from build123d import *

# Parameters (mm, degrees)
BOSS_EXTRUDE1_DEPTH = 36
BOSS_EXTRUDE2_DEPTH = 12
SKETCH1_6_W         = 12
SKETCH1_6_H         = 48
SKETCH1_6_W_2       = 25
SKETCH1_6_W_3       = 23
SKETCH1_6_H_2       = 12
BOSS_EXTRUDE4_DEPTH = 24
SKETCH1_8_W         = 25
SKETCH1_8_H         = 12
SKETCH1_8_H_2       = 48
SKETCH1_8_W_2       = 23
CUT_EXTRUDE2_DEPTH  = 12
BOSS_EXTRUDE5_START = 24
SKETCH1_10_W        = 23
SKETCH1_10_H        = 12
SKETCH1_10_W_2      = 12
SKETCH1_10_W_3      = 25
BOSS_EXTRUDE5_DEPTH = 12
CUT_EXTRUDE3_DEPTH  = 12
FILLET1_R           = 5


with BuildPart() as part:
    # Sketch1 → Boss-Extrude1 (new body)
    with BuildSketch(Plane(origin=(0, 0, 0), x_dir=(0, 1, 0), z_dir=(0, 0, 1))):
        with BuildLine():
            Line((36, -30), (27, -30))
            ThreePointArc((27, -30), (45, -48), (63, -30))
            ThreePointArc((63, -30), (57.727922061, -17.272077939), (45, -12))
            Line((45, -12), (45, -21))
            ThreePointArc((45, -21), (51.363961031, -23.636038969), (54, -30))
            ThreePointArc((54, -30), (45, -39), (36, -30))
        make_face()
        with BuildLine():
            ThreePointArc((39, -13.029437252), (30.303061543, -19.607695155), (27, -30))
            Line((27, -30), (36, -30))
            ThreePointArc((36, -30), (36.784161637, -26.325765386), (39, -23.291796068))
            Line((39, -23.291796068), (39, -13.029437252))
        make_face()
        with BuildLine():
            ThreePointArc((45, -12), (41.956164383, -12.259225926), (39, -13.029437252))
            Line((39, -13.029437252), (39, -23.291796068))
            ThreePointArc((39, -23.291796068), (41.788601192, -21.592448769), (45, -21))
            Line((45, -21), (45, -12))
        make_face()
        with BuildLine():
            ThreePointArc((39, 13.029437252), (30.303061543, 19.607695155), (27, 30))
            Line((27, 30), (27, 18))
            Line((27, 18), (27, -30))
            ThreePointArc((27, -30), (30.303061543, -19.607695155), (39, -13.029437252))
            Line((39, -13.029437252), (39, 13.029437252))
        make_face()
        with BuildLine():
            Line((36, 30), (27, 30))
            ThreePointArc((27, 30), (30.303061543, 19.607695155), (39, 13.029437252))
            Line((39, 13.029437252), (39, 23.291796068))
            ThreePointArc((39, 23.291796068), (36.784161637, 26.325765386), (36, 30))
        make_face()
        with BuildLine():
            ThreePointArc((63, 30), (45, 48), (27, 30))
            Line((27, 30), (36, 30))
            ThreePointArc((36, 30), (45, 39), (54, 30))
            ThreePointArc((54, 30), (51.363961031, 23.636038969), (45, 21))
            Line((45, 21), (45, 12))
            ThreePointArc((45, 12), (57.727922061, 17.272077939), (63, 30))
        make_face()
        with BuildLine():
            Line((39, 23.291796068), (39, 13.029437252))
            ThreePointArc((39, 13.029437252), (41.956164383, 12.259225926), (45, 12))
            Line((45, 12), (45, 21))
            ThreePointArc((45, 21), (41.788601192, 21.592448769), (39, 23.291796068))
        make_face()
    extrude(amount=BOSS_EXTRUDE1_DEPTH)

    # Sketch1_4 → Boss-Extrude2 (add)
    with BuildSketch(Plane(origin=(0, 0, 0), x_dir=(0, 1, 0), z_dir=(0, 0, 1))):
        with BuildLine():
            ThreePointArc((45, 12), (41.956164383, 12.259225926), (39, 13.029437252))
            Line((39, 13.029437252), (39, -13.029437252))
            ThreePointArc((39, -13.029437252), (41.956164383, -12.259225926), (45, -12))
            Line((45, -12), (45, 12))
        make_face()
        with BuildLine():
            Line((63, -30), (63, 30))
            ThreePointArc((63, 30), (57.727922061, 17.272077939), (45, 12))
            Line((45, 12), (45, -12))
            ThreePointArc((45, -12), (57.727922061, -17.272077939), (63, -30))
        make_face()
    extrude(amount=BOSS_EXTRUDE2_DEPTH)

    # Sketch1_6 → Boss-Extrude4 (add)
    # profile 1 of 8: a face of its own
    with BuildSketch(Plane(origin=(0, 0, 0), x_dir=(0, 1, 0), z_dir=(0, 0, 1))):
        with Locations((-2, -6)):
            Rectangle(SKETCH1_6_W, SKETCH1_6_H)
    # profile 2 of 8: a face of its own
    with BuildSketch(Plane(origin=(0, 0, 0), x_dir=(0, 1, 0), z_dir=(0, 0, 1))):
        with Locations((-20.5, -6)):
            Rectangle(SKETCH1_6_W_2, SKETCH1_6_H)
        with BuildLine():
            Line((-28, -8), (-28, 1))
            ThreePointArc((-28, 1), (-20, 9), (-12, 1))
            Line((-12, 1), (-12, -8))
            ThreePointArc((-12, -8), (-20, -16), (-28, -8))
        make_face(mode=Mode.SUBTRACT)
    # profile 3 of 8: a face of its own
    with BuildSketch(Plane(origin=(0, 0, 0), x_dir=(0, 1, 0), z_dir=(0, 0, 1))):
        with Locations((15.5, -6)):
            Rectangle(SKETCH1_6_W_3, SKETCH1_6_H)
    # profile 4 of 8: a face of its own
    with BuildSketch(Plane(origin=(0, 0, 0), x_dir=(0, 1, 0), z_dir=(0, 0, 1))):
        with Locations((-39, -6)):
            Rectangle(SKETCH1_6_W, SKETCH1_6_H)
    # profile 5 of 8: a face of its own
    with BuildSketch(Plane(origin=(0, 0, 0), x_dir=(0, 1, 0), z_dir=(0, 0, 1))):
        with Locations((15.5, 24)):
            Rectangle(SKETCH1_6_W_3, SKETCH1_6_H_2)
    # profile 6 of 8: a face of its own
    with BuildSketch(Plane(origin=(0, 0, 0), x_dir=(0, 1, 0), z_dir=(0, 0, 1))):
        with Locations((-2, 24)):
            Rectangle(SKETCH1_6_W, SKETCH1_6_H_2)
    # profile 7 of 8: a face of its own
    with BuildSketch(Plane(origin=(0, 0, 0), x_dir=(0, 1, 0), z_dir=(0, 0, 1))):
        with Locations((-20.5, 24)):
            Rectangle(SKETCH1_6_W_2, SKETCH1_6_H_2)
    # profile 8 of 8: a face of its own
    with BuildSketch(Plane(origin=(0, 0, 0), x_dir=(0, 1, 0), z_dir=(0, 0, 1))):
        with Locations((-39, 24)):
            Rectangle(SKETCH1_6_W, SKETCH1_6_H_2)
    extrude(amount=BOSS_EXTRUDE4_DEPTH)

    # Sketch1_8 → Cut-Extrude2 (cut)
    # profile 1 of 4: a face of its own
    with BuildSketch(Plane(origin=(0, 0, 0), x_dir=(0, 1, 0), z_dir=(0, 0, 1))):
        with Locations((-20.5, 24)):
            Rectangle(SKETCH1_8_W, SKETCH1_8_H)
    # profile 2 of 4: a face of its own
    with BuildSketch(Plane(origin=(0, 0, 0), x_dir=(0, 1, 0), z_dir=(0, 0, 1))):
        with Locations((-20.5, -6)):
            Rectangle(SKETCH1_8_W, SKETCH1_8_H_2)
        with BuildLine():
            Line((-28, -8), (-28, 1))
            ThreePointArc((-28, 1), (-20, 9), (-12, 1))
            Line((-12, 1), (-12, -8))
            ThreePointArc((-12, -8), (-20, -16), (-28, -8))
        make_face(mode=Mode.SUBTRACT)
    # profile 3 of 4: a face of its own
    with BuildSketch(Plane(origin=(0, 0, 0), x_dir=(0, 1, 0), z_dir=(0, 0, 1))):
        with Locations((15.5, 24)):
            Rectangle(SKETCH1_8_W_2, SKETCH1_8_H)
    # profile 4 of 4: a face of its own
    with BuildSketch(Plane(origin=(0, 0, 0), x_dir=(0, 1, 0), z_dir=(0, 0, 1))):
        with Locations((15.5, -6)):
            Rectangle(SKETCH1_8_W_2, SKETCH1_8_H_2)
    extrude(amount=CUT_EXTRUDE2_DEPTH, mode=Mode.SUBTRACT)

    # Sketch1_10 → Boss-Extrude5 (add)
    with BuildSketch(Plane(origin=(0, 0, 0), x_dir=(0, 1, 0), z_dir=(0, 0, 1)).offset(BOSS_EXTRUDE5_START)):
        with Locations((15.5, 24)):
            Rectangle(SKETCH1_10_W, SKETCH1_10_H)
        with Locations((-2, 24)):
            Rectangle(SKETCH1_10_W_2, SKETCH1_10_H)
        with Locations((-20.5, 24)):
            Rectangle(SKETCH1_10_W_3, SKETCH1_10_H)
        with Locations((-39, 24)):
            Rectangle(SKETCH1_10_W_2, SKETCH1_10_H)
    extrude(amount=BOSS_EXTRUDE5_DEPTH)

    # Sketch2 → Cut-Extrude3 (cut)
    with BuildSketch(Plane.YZ.offset(-18)):
        Polygon((-45, 24), (27, 36), (-45, 36), align=None)
    extrude(amount=-CUT_EXTRUDE3_DEPTH, mode=Mode.SUBTRACT)

    # Fillet1
    fillet1_edges = [part.edges().sort_by_distance(p)[0] for p in [
        (-13.029437252, 39, 24),
        (13.029437252, 39, 24),
    ]]
    fillet(fillet1_edges, radius=FILLET1_R)


solid = part.part
Can you work these out from the model? Positions are in its coordinate system, mm. A direction names the side the tool comes from. Give positions to 0.01 mm unless a question says otherwise; leave off trailing zeros. Write each loop counter-clockwise with the first axis right and the second up, starting at its lowest first coordinate (ties: lowest second). Pieces come first, ordered by that corner, then holes. Notation, with made-up numbers: (-18, 49) -> (-11, 49) arc R19 cw to (-11, 71) -> close; hole circle Ø3 at (-23, 22.25). An arc over 180 degrees is marked (long way). Answer as a JSON object with one key per item and string values. Group by question number.
Item 1: Suppose I cut it at C-C (y = -20). Please give me the cut outline in (x, z), plus the area to 3 significant figures.
Item 2: Suppose I cut it at A-A (z = 18). Please give me the cut outline in (x, y), plus the area to 3 significant figures.
Item 3: I'm going to push flat-ended pins straight in: P1, Ø12, axis at y = 12.5, z = 22, coming from the +X side; P2, Ø11, axis at x = -1, z = 30, coming from the +Y side; P3, Ø8, axis at x = 11.5, z = 24.5, coming from the +Y side. Where does each tip first touch, or does it pass through?
Item 4: We'd pull the mould along X, two halves only. Please class faces 4 (the face through (-30, -8, 18)), 5 (the face through (0, 53, 12)), 6 (the face through (0, -8, 6)): +X half, -X half, draft (parallel to the pull), parting line (faces both ways), or undercut.
Item 5: Please list where these lines run through material, in increasing order: line 1 (Y direction, x = 8.5, z = 3); line 2 (Y direction, x = 30.5, z = 20); line 3 (X direction, y = 41, z = 4). Write a range as [from, to].
Item 6: Suppose I cut it at B-B (z = 5.5). Please give me the cut outline in (x, y), plus the area to 3 significant figures.
Item 7: Suppose I cut it at D-D (x = 34.5). Please give me the cut outline in (y, z), plus the area to 3 significant figures.
Item 8: For faces 1 (the face through (-9, -20, 18)), 2 (the face through (0, 39, 24)), 3 (the face through (6, -10, 24)), which set-ups out of +Z, -Z, +X, -X, +Y, -Y let a thin tool reach every point of the face, with its end or its side?
Findings:
{
 "1": {"outline": "(-30, 12) -> (-9, 12) -> (-9, 24) -> (-18, 24) -> (-18, 28.17) -> (-30, 28.17) -> close; (16, 12) -> (30, 12) -> (30, 24) -> (16, 24) -> close", "area": "470 mm²"},
 "2": {"outline": "(-30, -45) -> (30, -45) -> (30, 27) arc R18 ccw (long way) to (12.02, 44.22) arc R5 cw to (7.02, 39) -> (-7.02, 39) arc R5 cw to (-12.02, 44.22) arc R18 ccw (long way) to (-30, 27) -> close; hole circle Ø18 at (-30, 45); hole (-1, -28) -> (8, -28) arc R8 ccw to (8, -12) -> (-1, -12) arc R8 ccw to start; hole circle Ø18 at (30, 45)", "area": "5,940 mm²"},
 "3": {"P1": "stops at x = 30", "P2": "stops at y = 39", "P3": "stops at y = 55.67"},
 "4": {"face 4": "-X half", "face 5": "undercut", "face 6": "draft"},
 "5": {"line 1": "y = [-45, -33], [-8, 4], [27, 63]", "line 2": "y = [27.01, 36.01], [53.99, 62.99]", "line 3": "x = [-47.55, -38.06], [-21.94, 21.94], [38.06, 47.55]"},
 "6": {"outline": "(-30, -45) -> (30, -45) -> (30, -33) -> (-30, -33) -> close; (-30, -8) -> (30, -8) -> (30, 4) -> (-30, 4) -> close; (-30, 27) -> (30, 27) arc R18 ccw to (30, 63) -> (-30, 63) arc R18 ccw to start; hole circle Ø18 at (-30, 45); hole circle Ø18 at (30, 45)", "area": "4,110 mm²"},
 "7": {"outline": "(27.57, 0) -> (37.21, 0) -> (37.21, 36) -> (27.57, 36) -> close; (52.79, 0) -> (62.43, 0) -> (62.43, 36) -> (52.79, 36) -> close", "area": "694 mm²"},
 "8": {"face 1": "+Z, -Z", "face 2": "+Z, +Y", "face 3": "+Z, +X, -Y"}
}
